For this review, use the dimensioned drawing (mm, ordinates from the lowest corner) and the shaded views. A direction names the side the tool comes from. Coordinates: 2 decimals unless noted, no trailing zeros. Loops run counter-clockwise (first coordinate to the right, second up) from the corner with the lowest first, then second, coordinate; pieces in that order, holes last.
1. Mouldability with a two-part tool opening along X and no side actions: class the marked faces 1, 2 and 3 as pulls with the +X half, pulls with the -X half, needs draft (parallel to the pull), parting line crosses it, or undercut.
2. Take a section at C-C, the plane x = 19. State the section outline as (y, z) points.
3. Take a section at B-B, the plane y = 20. State the section outline as (x, z) points.
4. To check wall thickness, follow probe 1 along Y at (x, z) = (19, 10.5); probe 2 along X at (y, z) = (6, 3.5); probe 3 along X at (y, z) = (12, 7.75) (1 decimal). State the ranges of each line that lie inside material, in increasing order.
5. Take a section at A-A, the plane x = 29.5. State the section outline as (y, z) points, then the cut area to 3 significant figures.
6. Take a section at D-D, the plane y = 34. State the section outline as (x, z) points.
7. Clearance check with flat-ended pins moving along their axes: P1, Ø6.5, axis at x = 48, z = 8.36, coming from the +Y side; P2, Ø1.8, axis at x = 59, y = 6, coming from the +Z side; P3, Ø5, axis at x = 5.5, z = 10.5, coming from the +Y side; P4, Ø5, axis at x = 48, z = 8, coming from the +Y side. State where each tip first meets the part, or that it passes through.
8. Machinability: for the marked faces 4, 5 and 6, which of the approach directions +Z, -Z, +X, -X, +Y, -Y give a long, thin tool a straight path to every point of the face, cutting with its end or side? Answer none if there is none.
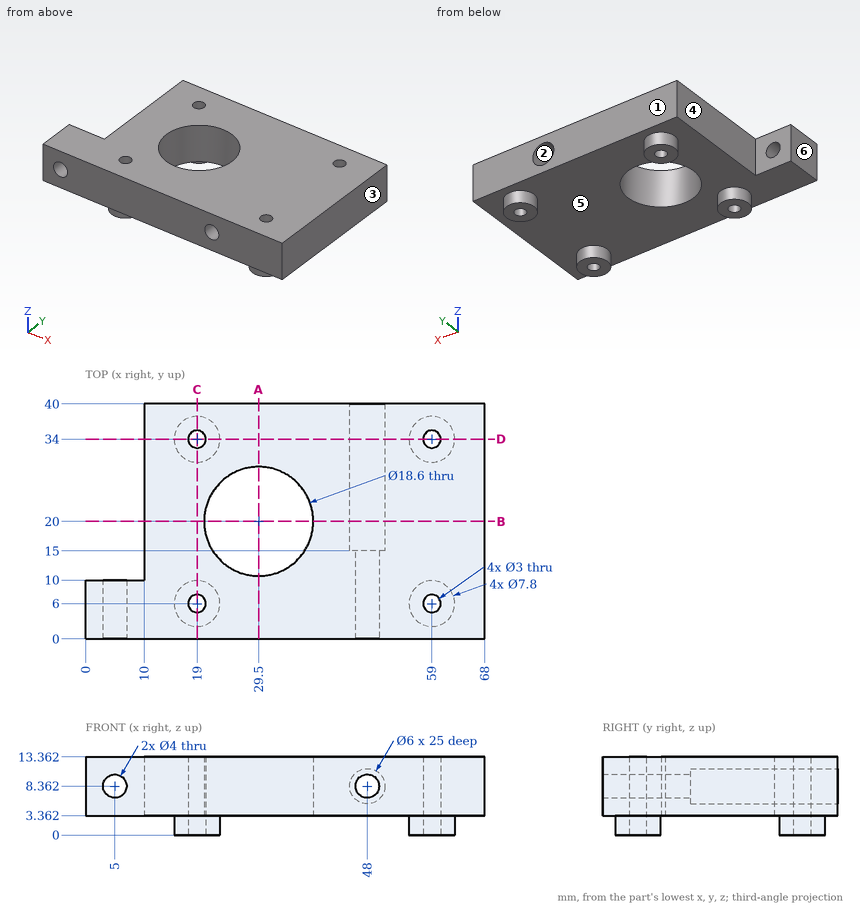
Results list:
1. face 1: needs draft
1. face 2: undercut
1. face 3: pulls with the +X half
2. outline: (0, 3.36) - (2.1, 3.36) - (2.1, 0) - (4.5, 0) - (4.5, 13.36) - (0, 13.36) - close; (7.5, 0) - (9.9, 0) - (9.9, 3.36) - (30.1, 3.36) - (30.1, 0) - (32.5, 0) - (32.5, 13.36) - (7.5, 13.36) - close; (35.5, 0) - (37.9, 0) - (37.9, 3.36) - (40, 3.36) - (40, 13.36) - (35.5, 13.36) - close
3. outline: (10, 3.36) - (20.2, 3.36) - (20.2, 13.36) - (10, 13.36) - close; (38.8, 3.36) - (68, 3.36) - (68, 13.36) - (38.8, 13.36) - close; hole circle Ø6 at (48, 8.36)
4. probe 1: y = 0 to 4.5, 7.5 to 32.5, 35.5 to 40
4. probe 2: x = 0 to 17.5, 20.5 to 57.5, 60.5 to 68
4. probe 3: x = 10 to 24.8, 34.2 to 46.1, 49.9 to 68
5. outline: (0, 3.36) - (10.7, 3.36) - (10.7, 13.36) - (0, 13.36) - close; (29.3, 3.36) - (40, 3.36) - (40, 13.36) - (29.3, 13.36) - close
5. area: 214 mm2
6. outline: (10, 3.36) - (15.1, 3.36) - (15.1, 0) - (17.5, 0) - (17.5, 13.36) - (10, 13.36) - close; (20.5, 0) - (22.9, 0) - (22.9, 3.36) - (55.1, 3.36) - (55.1, 0) - (57.5, 0) - (57.5, 13.36) - (20.5, 13.36) - close; (60.5, 0) - (62.9, 0) - (62.9, 3.36) - (68, 3.36) - (68, 13.36) - (60.5, 13.36) - close; hole circle Ø6 at (48, 8.36)
7. P1: stops at y = 40
7. P2: passes through
7. P3: stops at y = 10
7. P4: stops at y = 15
8. face 4: +Z, -Z, -X, +Y
8. face 5: -Z
8. face 6: +Z, -Z, -X, +Y, -Y
